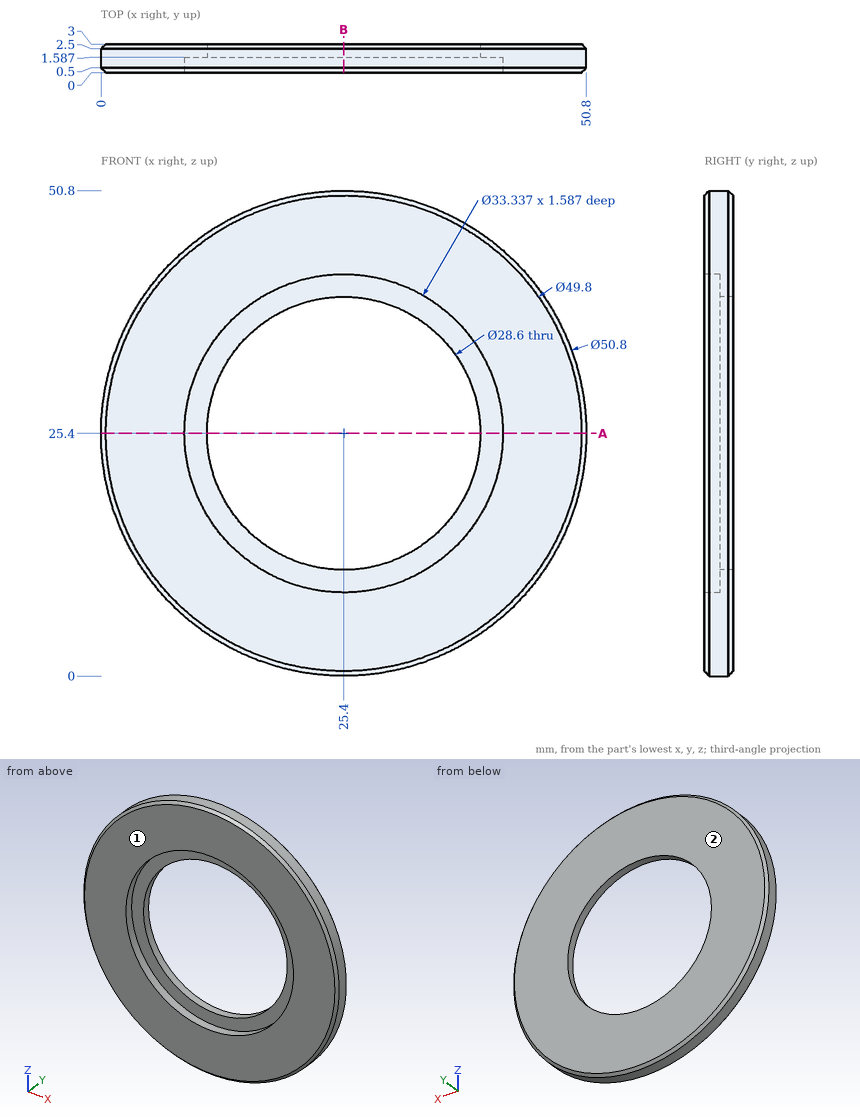
Input: dimensioned drawing with shaded views. Units: mm. Origin: part minimum x, y, z. Round coordinates to 2 decimals unless told otherwise and drop trailing zeros. Loops run counter-clockwise (first coordinate to the right, second up) from the corner with the lowest first, then second, coordinate; pieces in that order, holes last. Notation, with made-up numbers: (-23, 7) -> (9, 7) arc R8 ccw to (9, 16) -> close; hole circle Ø10 at (26, -27). An arc over 180 degrees is marked (long way). Use one line per item in the form item = value. Start each with the question number.
1) Section A-A on z = 25.4. Output: boundary loops of the cut face in (x, y).
2) Line query: L1, parallel to Z at x = 25.4, y = 1.1; L2, parallel to X at y = 0.5, z = 25 (1 decimal); L3, parallel to Z at x = 12, y = 0.2 (1 decimal). Output: solid intervals per line, ascending.
3) Section B-B on x = 25.4. Output: boundary loops of the cut face in (y, z).
4) First-contact query: P1, Ø10, axis at x = 31, z = 14.5, coming from the -Y side; P2, Ø1.5, axis at y = 2, z = 28, coming from the -X side. Flat tips, straight axial feed; report the tip coordinate or a pass-through.
5) Draft query along Y for the marked faces 1 and 2. Return one class per face: released by +Y, released by -Y, zero draft, split by the parting line, or undercut.
Response:
q1.outline = (0, 0.5) -> (0.5, 0) -> (8.73, 0) -> (8.73, 1.59) -> (11.1, 1.59) -> (11.1, 3) -> (0.5, 3) -> (0, 2.5) -> close; (39.7, 1.59) -> (42.07, 1.59) -> (42.07, 0) -> (50.3, 0) -> (50.8, 0.5) -> (50.8, 2.5) -> (50.3, 3) -> (39.7, 3) -> close
q2.L1 = 0 to 8.73, 42.07 to 50.8
q2.L2 = 0 to 8.7, 42.1 to 50.8
q2.L3 = 4.2 to 15.5, 35.3 to 46.6
q3.outline = (0, 0.5) -> (0.5, 0) -> (2.5, 0) -> (3, 0.5) -> (3, 11.1) -> (1.59, 11.1) -> (1.59, 8.73) -> (0, 8.73) -> close; (0, 42.07) -> (1.59, 42.07) -> (1.59, 39.7) -> (3, 39.7) -> (3, 50.3) -> (2.5, 50.8) -> (0.5, 50.8) -> (0, 50.3) -> close
q4.P1 = 0
q4.P2 = 0.07
q5.face_1 = released by -Y
q5.face_2 = released by +Y
